from build123d import *

# Parameters (mm, degrees)
SKETCH1_W                              = 296
SKETCH1_H                              = 196
SKETCH1_R                              = 13
SKETCH1_R_2                            = 3.5
SKETCH1_R_3                            = 6
SKETCH1_R_4                            = 5
EXTRUDE1_DEPTH                         = 36
CBORE_FOR_14_MM_CORE_PINS1_D           = 14
CBORE_FOR_14_MM_CORE_PINS1_CBORE_D     = 18
CBORE_FOR_14_MM_CORE_PINS1_CBORE_DEPTH = 5


with BuildPart() as part:
    # Sketch1 → Extrude1 (new body)
    with BuildSketch(Plane.XY):
        Rectangle(SKETCH1_W, SKETCH1_H)
        with Locations((-120, 75)):
            Circle(SKETCH1_R, mode=Mode.SUBTRACT)
        with Locations((-120, -75)):
            Circle(SKETCH1_R, mode=Mode.SUBTRACT)
        with Locations((120, 75)):
            Circle(SKETCH1_R, mode=Mode.SUBTRACT)
        with Locations((120, -75)):
            Circle(SKETCH1_R, mode=Mode.SUBTRACT)
        with Locations((-47, 10.939957651)):
            Circle(SKETCH1_R_2, mode=Mode.SUBTRACT)
        with Locations((-80, 10.939957651)):
            Circle(SKETCH1_R_2, mode=Mode.SUBTRACT)
        with Locations((-80, -10.939957651)):
            Circle(SKETCH1_R_2, mode=Mode.SUBTRACT)
        with Locations((-47, -10.939957651)):
            Circle(SKETCH1_R_2, mode=Mode.SUBTRACT)
        with Locations((47, -10.939957651)):
            Circle(SKETCH1_R_2, mode=Mode.SUBTRACT)
        with Locations((80, -10.939957651)):
            Circle(SKETCH1_R_2, mode=Mode.SUBTRACT)
        with Locations((80, 10.939957651)):
            Circle(SKETCH1_R_2, mode=Mode.SUBTRACT)
        with Locations((47, 10.939957651)):
            Circle(SKETCH1_R_2, mode=Mode.SUBTRACT)
        with Locations((-85, 36)):
            Circle(SKETCH1_R_3, mode=Mode.SUBTRACT)
        with Locations((-85, -36)):
            Circle(SKETCH1_R_3, mode=Mode.SUBTRACT)
        with Locations((85, 36)):
            Circle(SKETCH1_R_3, mode=Mode.SUBTRACT)
        with Locations((85, -36)):
            Circle(SKETCH1_R_3, mode=Mode.SUBTRACT)
        Circle(SKETCH1_R_4, mode=Mode.SUBTRACT)
    extrude(amount=-EXTRUDE1_DEPTH)

    # CBORE for 14 mm Core Pins1 (through all)
    with Locations(Plane.XY):
        with Locations((60, 30), (-60, 30), (-60, -30), (60, -30)):
            CounterBoreHole(CBORE_FOR_14_MM_CORE_PINS1_D / 2, CBORE_FOR_14_MM_CORE_PINS1_CBORE_D / 2, CBORE_FOR_14_MM_CORE_PINS1_CBORE_DEPTH)


solid = part.part
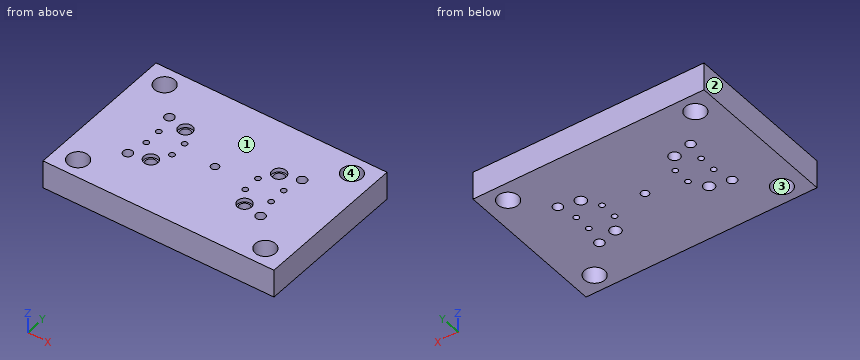
The model under review builds one solid part; all positions refer to its coordinate system, in mm. Face numbers are marked on the shaded views. Round coordinates to 2 decimals unless told otherwise and drop trailing zeros. Write each loop counter-clockwise with the first axis right and the second up, starting at its lowest first coordinate (ties: lowest second). Pieces come first, ordered by that corner, then holes. Notation, with made-up numbers: (81, 39) - (85, 39) arc R32 cw to (85, 73) - close; hole circle Ø2 at (46, 48.25). An arc over 180 degrees is marked (long way). One line per item, written item: value. Start each with the question number.
1. Consider section D-D on y = -75. Write out the cut boundary in (x, z), and give its area (3 significant figures).
2. Consider section A-A on x = 0. Write out the cut boundary in (y, z), and give its area (3 significant figures).
3. Clearance check with flat-ended pins moving along their axes: P1, Ø9, axis at x = -63.5, y = -28.5, coming from the +Z side; P2, Ø8, axis at x = 0, y = 0, coming from the +Z side; P3, Ø14, axis at x = -85, y = -36, coming from the +Z side. State where each tip first meets the part, or that it passes through.
4. The part is to be moulded in two halves that separate along X. For the marked faces 1, 2, 3 and 4, say which applies: released by +X, released by -X, zero draft, split by the parting line, or undercut.
5. Consider section B-B on x = 47. Write out the cut boundary in (y, z).
6. To check wall thickness, follow L1, parallel to Y at x = 60, z = -15; L2, parallel to Y at x = -60, z = -2.65; L3, parallel to X at y = 64.5, z = -7. State the ranges of each line that lie inside material, in increasing order. Write a range as from..to.
7. Consider section C-C on y = 0. Write out the cut boundary in (x, z).
Checks:
1. outline: (-148, -36) - (-133, -36) - (-133, 0) - (-148, 0) - close; (-107, -36) - (107, -36) - (107, 0) - (-107, 0) - close; (133, -36) - (148, -36) - (148, 0) - (133, 0) - close
1. area: 8,780 mm^2
2. outline: (-98, -36) - (-5, -36) - (-5, 0) - (-98, 0) - close; (5, -36) - (98, -36) - (98, 0) - (5, 0) - close
2. area: 6,700 mm^2
3. P1: stops at z = -5
3. P2: passes through
3. P3: stops at z = 0
4. face 1: zero draft
4. face 2: released by -X
4. face 3: undercut
4. face 4: undercut
5. outline: (-98, -36) - (-14.44, -36) - (-14.44, 0) - (-98, 0) - close; (-7.44, -36) - (7.44, -36) - (7.44, 0) - (-7.44, 0) - close; (14.44, -36) - (98, -36) - (98, 0) - (14.44, 0) - close
6. L1: y = -98..-37, -23..23, 37..98
6. L2: y = -98..-39, -21..21, 39..98
6. L3: x = -148..-127.66, -112.34..112.34, 127.66..148
7. outline: (-148, -36) - (-5, -36) - (-5, 0) - (-148, 0) - close; (5, -36) - (148, -36) - (148, 0) - (5, 0) - close
